```python
from build123d import *

# Parameters (mm, degrees)
BOSS_EXTRUDE1_DEPTH = 11
SKETCH3_R           = 1.2
SKETCH3_W           = 5.5
SKETCH3_H           = 4.5
CUT_EXTRUDE1_DEPTH  = 22.508661046


with BuildPart() as part:
    # Sketch1 → Boss-Extrude1 (new body)
    with BuildSketch(Plane(origin=(0, 0, 0), x_dir=(0, 0, -1), z_dir=(1, 0, 0))):
        Polygon((0, 0), (-2.95, 0), (-2.95, 18.4), (0, 18.4), (0, 17.2), (-1.75, 17.2), (-1.75, 1.2), (0, 1.2), align=None)
    extrude(amount=BOSS_EXTRUDE1_DEPTH)

    # Sketch3 → Cut-Extrude1 (cut, through all)
    with BuildSketch(Plane(origin=(0, 0, 1.75), x_dir=(-1, 0, 0), z_dir=(0, 0, -1))):
        with Locations(Location((-9, 15.2, 0), (0, 0, 90))):
            Circle(SKETCH3_R)
        with Locations(Location((-2, 3.2, 0), (0, 0, 90))):
            Circle(SKETCH3_R)
        with Locations((-2.75, 10.45)):
            Rectangle(SKETCH3_W, SKETCH3_H)
    extrude(amount=-CUT_EXTRUDE1_DEPTH, mode=Mode.SUBTRACT)


solid = part.part
```
Could you check a few things on this model? Use its own coordinates, in mm. A direction names the side the tool comes from. Round coordinates to 2 decimals unless told otherwise and drop trailing zeros. Write each loop counter-clockwise with the first axis right and the second up, starting at its lowest first coordinate (ties: lowest second). Pieces come first, ordered by that corner, then holes. Notation, with made-up numbers: M 55.25,-18.75 L 104.25,-18.75 A21 ccw 104.25,6.25 Z; hole C -6.75,52 d8. An arc over 180 degrees is marked long. Answer in a Markdown table with one row per item. Add a question column.
Q1. Imagine slicing it at D-D (x = 9). Please give me the cut outline in (y, z), then the cut area to 3 significant figures.
Q2. If we mould it in two halves opening along Y, with no side actions, what happens to faces 4 (the flat face through (5, 18, 0)), 5 (the flat face through (5.5, 10, 2)), 6 (the flat face through (5, 0, 1))? For each: +Y half, -Y half, draft (parallel to the pull), parting line (faces both ways), or undercut.
Q3. If I drill on line 1 (Y direction, x = 3.25, z = 1.1); line 2 (Y direction, x = 3.75, z = 2.2); line 3 (X direction, y = 3.2, z = 2.25), over which ranges is the centre line in solid material (lowest first)? Write a range as from..to.
Q4. On a 3-axis mill with a long thin cutter (end or side, diameter ignored), from which of +Z, -Z, +X, -X, +Y, -Y can I reach the whole of each face in a straight line? I mean faces 1 (the flat face through (5, 1.2, 1)), 2 (the flat face through (3, 8.2, 2)), 3 (the flat face through (0, 16, 2)). Say none if no direction works.
Q5. Imagine slicing it at C-C (y = 15.2). Please give me the cut outline in (x, z), then the cut area to 3 significant figures.
Q6. Imagine slicing it at B-B (x = 2). Please give me the cut outline in (y, z), then the cut area to 3 significant figures.
Q7. Will these pins go through, and if not, where does the flat tip stop? pin 1 Ø4 at (x, y) = (6.5, 5) entering from -Z; pin 2 Ø1 at (y, z) = (10, 2.5) entering from -X.
Q8. Imagine slicing it at A-A (z = 2.6). Please give me the cut outline in (x, y).
Values:
| question | item | result |
|---|---|---|
| 1 | outline | M 0,0 L 1.2,0 L 1.2,1.75 L 14,1.75 L 14,2.95 L 0,2.95 Z; M 16.4,1.75 L 17.2,1.75 L 17.2,0 L 18.4,0 L 18.4,2.95 L 16.4,2.95 Z |
| 1 | area | 23.4 mm^2 |
| 2 | face 4 | draft |
| 2 | face 5 | undercut |
| 2 | face 6 | -Y half |
| 3 | line 1 | 0..1.2, 17.2..18.4 |
| 3 | line 2 | 0..8.2, 12.7..18.4 |
| 3 | line 3 | 0..0.8, 3.2..11 |
| 4 | face 1 | -Z, +X, -X |
| 4 | face 2 | +Z, -Z, -X |
| 4 | face 3 | +Z, -Z, -X, +Y, -Y |
| 5 | outline | M 0,1.75 L 7.8,1.75 L 7.8,2.95 L 0,2.95 Z; M 10.2,1.75 L 11,1.75 L 11,2.95 L 10.2,2.95 Z |
| 5 | area | 10.3 mm^2 |
| 6 | outline | M 0,0 L 1.2,0 L 1.2,1.75 L 2,1.75 L 2,2.95 L 0,2.95 Z; M 4.4,1.75 L 8.2,1.75 L 8.2,2.95 L 4.4,2.95 Z; M 12.7,1.75 L 17.2,1.75 L 17.2,0 L 18.4,0 L 18.4,2.95 L 12.7,2.95 Z |
| 6 | area | 18.0 mm^2 |
| 7 | pin 1 | z = 1.75 |
| 7 | pin 2 | x = 5.5 |
| 8 | outline | M 0,0 L 11,0 L 11,18.4 L 0,18.4 L 0,12.7 L 5.5,12.7 L 5.5,8.2 L 0,8.2 Z; hole C 2,3.2 d2.4; hole C 9,15.2 d2.4 |
